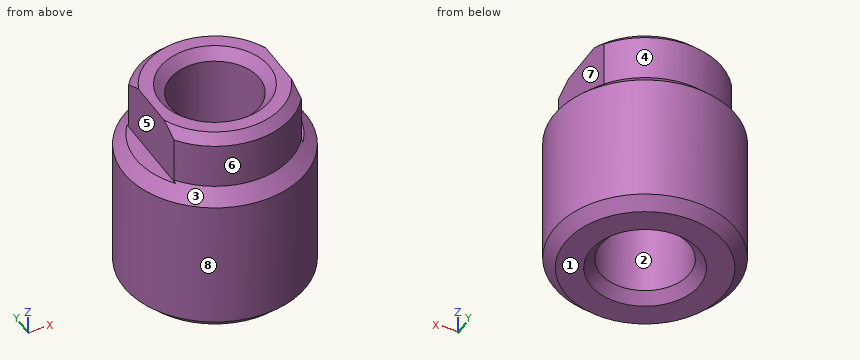
```python
from build123d import *

# Parameters (mm, degrees)
SCHNITT_LINEAR_AUSTRAGEN1_DEPTH      = 30
SCHNITT_LINEAR_AUSTRAGEN1_DEPTH_BACK = 30


with BuildPart() as part:
    # Skizze1 → Rotation1 (revolve)
    with BuildSketch(Plane(origin=(0, 0, 0), x_dir=(0, 0, -1), z_dir=(1, 0, 0))):
        Polygon((-11.5, 3.75), (-11.5, 3), (-10.9585, 2.4585), (-0.5415, 2.4585), (0, 3), (0, 4.3865), (-0.6135, 5), (-7.75, 5), (-8.5, 4.25), (-11, 4.25), align=None)
    revolve(axis=Axis((0, 0, 0), (0, 0, 1)))

    # Skizze2 → Schnitt-Linear austragen1 (cut, two sides)
    with BuildSketch(Plane(origin=(0, 0, 0), x_dir=(1, 0, 0), z_dir=(0, 1, 0))) as schnitt_linear_austragen1_sk:
        Polygon((-13.5, -23.4), (13.5, -23.4), (13.5, -8.4), (3.5, -8.4), (3.5, -18.4), (-3.5, -18.4), (-3.5, -8.4), (-13.5, -8.4), align=None)
    extrude(amount=SCHNITT_LINEAR_AUSTRAGEN1_DEPTH, mode=Mode.SUBTRACT)
    extrude(schnitt_linear_austragen1_sk.sketch, amount=-SCHNITT_LINEAR_AUSTRAGEN1_DEPTH_BACK, mode=Mode.SUBTRACT)


solid = part.part
```
Input: part model. Units: mm. Frame: model coordinates. Face numbers are marked on the shaded views. A direction names the side the tool comes from. Give positions to 0.01 mm unless a question says otherwise; leave off trailing zeros. Order: outer loops, then holes, each group sorted by start corner. A loop starts at its lowest first (then second) coordinate and runs counter-clockwise, first axis right, second up.
1. Section B-B on y = 0. Return the cut outline in (x, z).
Derived:
outline: (-5, 0.61) - (-4.39, 0) - (-3, 0) - (-2.46, 0.54) - (-2.46, 10.96) - (-3, 11.5) - (-3.5, 11.5) - (-3.5, 8.4) - (-4.35, 8.4) - (-5, 7.75) - close; (2.46, 0.54) - (3, 0) - (4.39, 0) - (5, 0.61) - (5, 7.75) - (4.35, 8.4) - (3.5, 8.4) - (3.5, 11.5) - (3, 11.5) - (2.46, 10.96) - close
2. Pin query (flat end, axial travel): pin 1 (5.5 mm diameter, centred on x = 0, y = 0, fed in from +Z); pin 2 (3 mm diameter, centred on x = -1, y = 1, fed in from +Z); pin 3 (1.5 mm diameter, centred on y = -0.5, z = 9, fed in from -X). Return the tip coordinate at first contact, or that it passes through.
Derived:
pin 1: stops at z = 11.25
pin 2: stops at z = 11.41
pin 3: stops at x = -4.48
3. Reachability of the marked faces 4, 5, 6, 7 and 8 from +Z, -Z, +X, -X, +Y, -Y: full face, straight path, thin tool, end or side. Return the list, or none.
Derived:
face 4: +Z, +Y
face 5: +Z, -X, +Y, -Y
face 6: +Z, -Y
face 7: +Z, +X, +Y, -Y
face 8: +Z, -Z
4. Section A-A on x = 0. Return the cut outline in (y, z), and give its area (3 significant figures).
Derived:
outline: (-5, 0.61) - (-4.39, 0) - (-3, 0) - (-2.46, 0.54) - (-2.46, 10.96) - (-3, 11.5) - (-3.75, 11.5) - (-4.25, 11) - (-4.25, 8.5) - (-5, 7.75) - close; (2.46, 0.54) - (3, 0) - (4.39, 0) - (5, 0.61) - (5, 7.75) - (4.25, 8.5) - (4.25, 11) - (3.75, 11.5) - (3, 11.5) - (2.46, 10.96) - close
area: 52.2 mm2
5. Material intervals for L1, parallel to Y at x = 0, z = 6.5; L2, parallel to X at y = 1.25, z = 4, sorted ascending.
Derived:
L1: y = -5 to -2.46, 2.46 to 5
L2: x = -4.84 to -2.12, 2.12 to 4.84
6. Section C-C on z = 5. Return the cut outline in (x, y), and give its area (3 significant figures).
Derived:
outline: circle Ø10 at (0, 0); hole circle Ø4.92 at (0, 0)
area: 59.6 mm2
7. Mould query, pull axis Y, two halves, no side actions, for the marked faces 1, 2 and 3. Classes: released by +Y, released by -Y, zero draft, split by the parting line, or undercut.
Derived:
face 1: zero draft
face 2: undercut
face 3: split by the parting line
